Autodesk Inventor part; units mm, degrees
ref_plane "YZ Plane" through (0, 0, 0) normal (1, 0, 0) x (0, 1, 0)
ref_plane "XZ Plane" through (0, 0, 0) normal (0, 1, 0) x (-1, 0, 0)
ref_plane "XY Plane" through (0, 0, 0) normal (0, 0, 1) x (1, 0, 0)
sketch "Esquisse1" plane through (0, 0, 0) normal (0, 1, 0) x (-1, 0, 0)
  line L0 (230, 200) -> (-230, 200)
  line L1 (-230, 200) -> (-230, -200)
  line L2 (-230, -200) -> (230, -200)
  line L3 (230, -200) -> (230, 200)
  point P0 (0, 0)
  dimension "d0" = 400
  dimension "d1" = 460
  dimension "d2" = 230
  dimension "d3" = 200
extrude "Extrusion1" add sketch "Esquisse1" along normal blind 30
sketch "Esquisse2" plane through (0, 0, 0) normal (0, -1, 0) x (1, 0, 0)
  circle A0 centre (215, 185) radius 15
  circle A1 centre (215, -185) radius 15
  circle A2 centre (-215, -185) radius 15
  circle A3 centre (-215, 185) radius 15
  line L0 (-230, 200) -> (230, 200)
  line L1 (230, 200) -> (230, -200)
  line L2 (230, -200) -> (-230, -200)
  line L3 (-230, -200) -> (-230, 200)
  point P0 (0, 0)
  dimension "d6" = 30
  dimension "d7" = 30
  dimension "d8" = 30
  dimension "d9" = 30
  dimension "d10" = 15
  dimension "d11" = 15
  dimension "d12" = 15
  dimension "d13" = 15
  dimension "d14" = 15
  dimension "d15" = 15
  dimension "d16" = 15
  dimension "d17" = 15
extrude "Extrusion2" add sketch "Esquisse2" along normal blind 410 contours A0 | A1 | A3 | A2
sketch "Esquisse3" plane through (0, 30, 0) normal (0, 1, 0) x (1, 0, 0)
  arc A0 (-215, -200) -> (-230, -185) centre (-215, -185) ccw
  circle A1 centre (-215, -185) radius 15
  arc A2 (-230, 185) -> (-215, 200) centre (-215, 185) ccw
  circle A3 centre (-215, 185) radius 15
  point P0 (0, 0)
extrude "Extrusion3" add sketch "Esquisse3" along normal blind 160
sketch "Esquisse4" plane through (-215, 190, 185) normal (0, 1, 0) x (1, 0, 0)
  line L0 (430, 385) -> (0, 385)
  line L1 (-15, -15) -> (18, -15)
  line L2 (18, -15) -> (18, 385)
  line L3 (18, 385) -> (-15, 385)
  line L4 (-15, 385) -> (-15, -15)
  point P0 (215, 185)
  dimension "d22" = 33
extrude "Extrusion4" add sketch "Esquisse4" along normal blind 200
equation "\"d7\" = d6"
equation "\"d8\" = d6"
equation "\"d9\" = d6"
equation "\"d12\" = d11"
equation "\"d13\" = d10"
equation "\"d14\" = d11"
equation "\"d15\" = d11"
equation "\"d16\" = d11"
equation "\"d17\" = d11"
properties part number "Chaise"
Model file for the job. Use its own axes, mm. A direction names the side the tool comes from. Round coordinates to 2 decimals unless told otherwise and drop trailing zeros. Loops run counter-clockwise (first coordinate to the right, second up) from the corner with the lowest first, then second, coordinate; pieces in that order, holes last. Notation, with made-up numbers: (-7.75, -9.75) - (24.25, -9.75) arc R16 cw to (24.25, 11.25) - close; hole circle Ø9 at (16.5, -14). An arc over 180 degrees is marked (long way). Write each question's results on one line, items separated by ' | '.
(1) Saw through at D-D, the plane y = 217.5. List the corners of the cut face in (x, z), then the cut area to 3 significant figures.
Answer below:
outline: (-230, -200) - (-197, -200) - (-197, 200) - (-230, 200) - close | area: 13,200 mm^2
(2) Wall check: L1, parallel to Y at x = -115.5, z = -31; L2, parallel to Y at x = -210.5, z = 102; L3, parallel to X at y = 191, z = -6.5. Give the ranges that are in metal, low to high.
Answer below:
L1: y = 0 to 30 | L2: y = 0 to 30, 190 to 390 | L3: x = -230 to -197
(3) Saw through at B-B, the plane y = -184. List the corners of the cut face in (x, z).
Answer below:
outline: circle Ø30 at (-215, -185); circle Ø30 at (-215, 185); circle Ø30 at (215, -185); circle Ø30 at (215, 185)
(4) Mould opens along X. For faces 4 (the flat face through (-214, 390, -3)), 5 (the cylindrical face through (-208.08, -202.13, 198.31)), 6 (the flat face through (-230, 289, -3)) say: released by +X, released by -X, zero draft, split by the parting line, or undercut.
Answer below:
face 4: zero draft | face 5: undercut | face 6: released by -X
(5) Saw through at A-A, the plane z = 28. List the corners of the cut face in (x, y).
Answer below:
outline: (-230, 0) - (230, 0) - (230, 30) - (-230, 30) - close; (-230, 190) - (-197, 190) - (-197, 390) - (-230, 390) - close
(6) Pin check, flat tips, straight feed: pin 1 (6 mm diameter, centred on x = 74.5, z = -89.5, fed in from +Y); pin 2 (10 mm diameter, centred on x = 179.5, z = 50.5, fed in from -Y). Stop position of each tip, or through.
Answer below:
pin 1: stops at y = 30 | pin 2: stops at y = 0
(7) 3-axis set-ups, long thin cutter, end or side, ignore diameter. For faces 1 (the cylindrical face through (221.92, -202.13, -171.69)), 2 (the flat face through (215, -410, -185)), 3 (the cylindrical face through (-200.357, 108.88, 181.748)): which of +Z, -Z, +X, -X, +Y, -Y reach the whole face in a straight line?
Answer below:
face 1: -Y | face 2: +Z, -Z, +X, -X, -Y | face 3: none
(8) Saw through at C-C, the plane x = 124.5. List the corners of the cut face in (y, z), then the cut area to 3 significant figures.
Answer below:
outline: (0, -200) - (30, -200) - (30, 200) - (0, 200) - close | area: 12,000 mm^2
